Autodesk Fusion 360 part; units mm, degrees
sketch "Sketch1" plane through (0, 0, 0) normal (0, 0, 1) x (1, 0, 0)
  line L0 (34.65, 25.65) -> (-34.65, 25.65)
  line L1 (-34.65, 25.65) -> (-34.65, -25.65)
  line L2 (-34.65, -25.65) -> (34.65, -25.65)
  line L3 (34.65, -25.65) -> (34.65, 25.65)
  line L4 (34.65, 25.65) -> (-34.65, -25.65) construction
  line L5 (-34.65, 25.65) -> (34.65, -25.65) construction
  dimension "d1" = 69.3
  dimension "d2" = 51.3
extrude "Extrude1" add sketch "Sketch1" along normal blind 2
sketch "Sketch2" plane through (0, 0, 2) normal (0, 0, 1) x (-1, 0, 0)
  line L0 (-34.65, 25.65) -> (-34.65, -25.65)
  line L1 (-34.65, -25.65) -> (34.65, -25.65)
  line L2 (34.65, -25.65) -> (34.65, 25.65)
  line L3 (34.65, 25.65) -> (-34.65, 25.65)
  line L4 (34.65, -25.65) -> (29.65, -25.65)
  line L5 (29.65, -25.65) -> (29.65, -30.65)
  line L6 (29.65, -30.65) -> (34.65, -30.65)
  line L7 (34.65, -30.65) -> (34.65, -25.65)
  line L8 (-34.65, -25.65) -> (-29.65, -25.65)
  line L9 (-29.65, -25.65) -> (-29.65, -30.65)
  line L10 (-29.65, -30.65) -> (-34.65, -30.65)
  line L11 (-34.65, -30.65) -> (-34.65, -25.65)
  line L12 (34.65, 25.65) -> (29.65, 25.65)
  line L13 (29.65, 25.65) -> (29.65, 30.65)
  line L14 (29.65, 30.65) -> (34.65, 30.65)
  line L15 (34.65, 30.65) -> (34.65, 25.65)
  line L16 (-34.65, 25.65) -> (-29.65, 25.65)
  line L17 (-29.65, 25.65) -> (-29.65, 30.65)
  line L18 (-29.65, 30.65) -> (-34.65, 30.65)
  line L19 (-34.65, 30.65) -> (-34.65, 25.65)
  dimension "d5" = 5
  dimension "d6" = 5
  dimension "d7" = 5
  dimension "d8" = 5
  dimension "d9" = 5
  dimension "d10" = 5
  dimension "d11" = 5
  dimension "d12" = 5
extrude "Extrude2" add sketch "Sketch2" along normal blind 5 from surface at -2 contours L3 L16 L17 L18 L19 | L1 L8 L9 L10 L11 | L3 L12 L13 L14 L15 | L1 L4 L5 L6 L7
sketch "Sketch3" plane through (0, 0, 0) normal (0, 0, -1) x (1, 0, 0)
  line L0 (34.65, -30.65) -> (34.65, 30.65)
  line L1 (34.65, 30.65) -> (29.65, 30.65)
  line L2 (29.65, 30.65) -> (29.65, 25.65)
  line L3 (29.65, 25.65) -> (-29.65, 25.65)
  line L4 (-29.65, 25.65) -> (-29.65, 30.65)
  line L5 (-29.65, 30.65) -> (-34.65, 30.65)
  line L6 (-34.65, 30.65) -> (-34.65, -30.65)
  line L7 (-34.65, -30.65) -> (-29.65, -30.65)
  line L8 (-29.65, -30.65) -> (-29.65, -25.65)
  line L9 (-29.65, -25.65) -> (29.65, -25.65)
  line L10 (29.65, -25.65) -> (29.65, -30.65)
  line L11 (29.65, -30.65) -> (34.65, -30.65)
  circle A0 centre (-32.15, 28.15) radius 1.6
  circle A1 centre (32.15, 28.15) radius 1.6
  circle A2 centre (32.15, -28.15) radius 1.6
  circle A3 centre (-32.15, -28.15) radius 1.6
  dimension "d16" = 3.2
  dimension "d17" = 3.2
  dimension "d18" = 3.2
  dimension "d19" = 3.2
  dimension "d20" = 2.5
  dimension "d21" = 2.5
  dimension "d22" = 2.5
  dimension "d23" = 2.5
  dimension "d24" = 2.5
  dimension "d25" = 2.5
  dimension "d26" = 2.5
  dimension "d27" = 2.5
extrude "Extrude3" cut sketch "Sketch3" against normal blind 3.1 contours A0 | A1 | A2 | A3
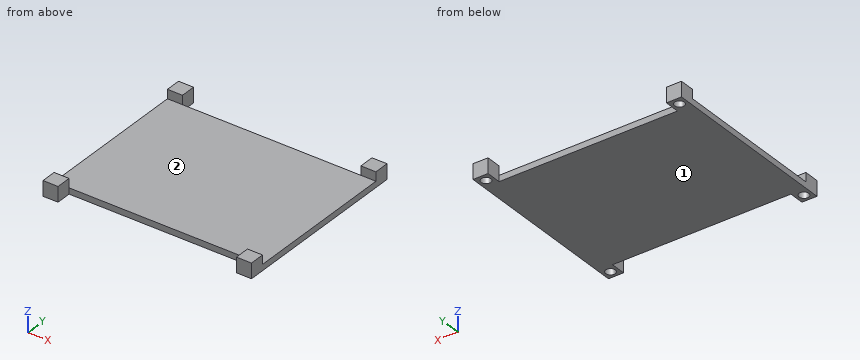
Part model, mm, in its own coordinate system. Face numbers are marked on the shaded views. Round coordinates to 2 decimals unless told otherwise and drop trailing zeros. Order: outer loops, then holes, each group sorted by start corner. A loop starts at its lowest first (then second) coordinate and runs counter-clockwise, first axis right, second up. Notation, with made-up numbers: M -32,-16.75 L -19,-16.75 A27 ccw -19,22.25 Z; hole C -6.5,-13.75 d6. An arc over 180 degrees is marked long. Answer in a Markdown table with one row per item. Add a question column.
Q1. Pin check, flat tips, straight feed: pin 1 (6 mm diameter, centred on x = -12.5, y = -18, fed in from +Z); pin 2 (0.6 mm diameter, centred on x = 13, z = 1, fed in from -Y); pin 3 (6 mm diameter, centred on x = -18, y = 22.5, fed in from -Z); pin 4 (1 mm diameter, centred on x = 31.5, y = -28.5, fed in from -Z). Stop position of each tip, or through.
Q2. Cut at A-A on z = 4.05. Give the cut face in (x, y), and give its area (3 significant figures).
Q3. Cut at B-B on y = -28.15. Give the cut face in (x, z).
Q4. Cut at C-C on x = 32.15. Give the cut face in (y, z).
Q5. Wall check: L1, parallel to Y at x = -32.15, z = 1.65; L2, parallel to Y at x = 32.15, z = 2.4; L3, parallel to X at y = 28.15, z = 2.45. Give the ranges that are in metal, low to high. Write a range as from..to.
Q6. Mould opens along Y. For the marked faces 1 and 2 say: +Y half, -Y half, draft (parallel to the pull), parting line (faces both ways), or undercut.
Q7. Cut at D-D on y = 23. Give the cut face in (x, z), and give its area (3 significant figures).
Established:
| question | item | result |
|---|---|---|
| 1 | pin 1 | stops at z = 2 |
| 1 | pin 2 | stops at y = -25.65 |
| 1 | pin 3 | stops at z = 0 |
| 1 | pin 4 | stops at z = 3.1 |
| 2 | outline | M -34.65,-30.65 L -29.65,-30.65 L -29.65,-25.65 L -34.65,-25.65 Z; M -34.65,25.65 L -29.65,25.65 L -29.65,30.65 L -34.65,30.65 Z; M 29.65,-30.65 L 34.65,-30.65 L 34.65,-25.65 L 29.65,-25.65 Z; M 29.65,25.65 L 34.65,25.65 L 34.65,30.65 L 29.65,30.65 Z |
| 2 | area | 100 mm2 |
| 3 | outline | M -34.65,0 L -33.75,0 L -33.75,3.1 L -30.55,3.1 L -30.55,0 L -29.65,0 L -29.65,5 L -34.65,5 Z; M 29.65,0 L 30.55,0 L 30.55,3.1 L 33.75,3.1 L 33.75,0 L 34.65,0 L 34.65,5 L 29.65,5 Z |
| 4 | outline | M -30.65,0 L -29.75,0 L -29.75,3.1 L -26.55,3.1 L -26.55,0 L 26.55,0 L 26.55,3.1 L 29.75,3.1 L 29.75,0 L 30.65,0 L 30.65,5 L 25.65,5 L 25.65,2 L -25.65,2 L -25.65,5 L -30.65,5 Z |
| 5 | L1 | y = -30.65..-29.75, -26.55..26.55, 29.75..30.65 |
| 5 | L2 | y = -30.65..-29.75, -26.55..-25.65, 25.65..26.55, 29.75..30.65 |
| 5 | L3 | x = -34.65..-33.75, -30.55..-29.65, 29.65..30.55, 33.75..34.65 |
| 6 | face 1 | draft |
| 6 | face 2 | undercut |
| 7 | outline | M -34.65,0 L 34.65,0 L 34.65,2 L -34.65,2 Z |
| 7 | area | 139 mm2 |
